```python
from build123d import *

# Parameters (mm, degrees)
BOSS_EXTRUDE1_DEPTH   = 1.5875
SKETCH3_R             = 4.445
SKETCH3_W             = 12.065
SKETCH3_H             = 12.065
CUT_EXTRUDE1_DEPTH    = 2.5875
SKETCH4_R             = 3.96875
CUT_EXTRUDE2_DEPTH    = 2.5875
SKETCH5_W             = 11.94
SKETCH5_H             = 20.64
SKETCH5_W_2           = 45.462
SKETCH5_H_2           = 102.32
SKETCH5_W_3           = 57
SKETCH5_H_3           = 15.1
CUT_EXTRUDE3_DEPTH    = 2.5875
F_6_CLEARANCE_HOLE2_D = 4.3053
CUT_EXTRUDE4_START    = -1.5875
SKETCH11_W            = 13.529020254
SKETCH11_H            = 14.424558238
SKETCH11_W_2          = 13.332833864
SKETCH11_H_2          = 14.312726797
CUT_EXTRUDE4_DEPTH    = 1.5875


with BuildPart() as part:
    # Sketch1 → Boss-Extrude1 (new body)
    with BuildSketch(Plane.XY):
        with BuildLine():
            Line((74.93, -171.1167297), (86.51875, -171.1167297))
            Line((86.51875, -171.1167297), (86.51875, -67.9292297))
            Line((86.51875, -67.9292297), (-86.51875, -67.9292297))
            Line((-86.51875, -67.9292297), (-86.51875, -171.1167297))
            Line((-86.51875, -171.1167297), (-74.93, -171.1167297))
            ThreePointArc((-74.93, -171.1167297), (-71.337897552, -172.604627251), (-69.85, -176.1967297))
            Line((-69.85, -176.1967297), (-69.85, -182.2292297))
            Line((-69.85, -182.2292297), (69.85, -182.2292297))
            Line((69.85, -182.2292297), (69.85, -176.1967297))
            ThreePointArc((69.85, -176.1967297), (71.337897552, -172.604627251), (74.93, -171.1167297))
        make_face()
    extrude(amount=-BOSS_EXTRUDE1_DEPTH)

    # Sketch3 → Cut-Extrude1 (cut, through all)
    with BuildSketch(Plane.XY):
        with Locations((74.93, -159.3692297)):
            Circle(SKETCH3_R)
        with Locations((-6.731, -165.7192297)):
            Circle(SKETCH3_R)
        with Locations((-6.731, -145.3992297)):
            Circle(SKETCH3_R)
        with Locations((-6.731, -125.0792297)):
            Circle(SKETCH3_R)
        with Locations((-6.731, -104.7592297)):
            Circle(SKETCH3_R)
        with Locations((-6.731, -84.4392297)):
            Circle(SKETCH3_R)
        with Locations((-73.66, -139.0492297)):
            Rectangle(SKETCH3_W, SKETCH3_H)
        with Locations((13.843, -143.3672297)):
            Rectangle(SKETCH3_W, SKETCH3_H)
        with Locations((32.639, -143.3672297)):
            Rectangle(SKETCH3_W, SKETCH3_H)
        with Locations((51.435, -143.3672297)):
            Rectangle(SKETCH3_W, SKETCH3_H)
        with Locations((51.435, -124.5712297)):
            Rectangle(SKETCH3_W, SKETCH3_H)
        with Locations((32.639, -124.5712297)):
            Rectangle(SKETCH3_W, SKETCH3_H)
        with Locations((13.843, -124.5712297)):
            Rectangle(SKETCH3_W, SKETCH3_H)
        with Locations((13.843, -105.7752297)):
            Rectangle(SKETCH3_W, SKETCH3_H)
        with Locations((13.843, -86.9792297)):
            Rectangle(SKETCH3_W, SKETCH3_H)
        with Locations((32.639, -86.9792297)):
            Rectangle(SKETCH3_W, SKETCH3_H)
        with Locations((32.639, -105.7752297)):
            Rectangle(SKETCH3_W, SKETCH3_H)
        with Locations((51.435, -105.7752297)):
            Rectangle(SKETCH3_W, SKETCH3_H)
        with Locations((51.435, -86.9792297)):
            Rectangle(SKETCH3_W, SKETCH3_H)
    extrude(amount=-CUT_EXTRUDE1_DEPTH, mode=Mode.SUBTRACT)

    # Sketch4 → Cut-Extrude2 (cut, through all)
    with BuildSketch(Plane.XY):
        with Locations((-73.025, -113.9667297)):
            Circle(SKETCH4_R)
        with Locations((-73.025, -159.0517297)):
            Circle(SKETCH4_R)
        with Locations((74.295, -113.9667297)):
            Circle(SKETCH4_R)
        with Locations((75.184, -139.0492297)):
            Circle(SKETCH4_R)
    extrude(amount=-CUT_EXTRUDE2_DEPTH, mode=Mode.SUBTRACT)

    # Sketch5 → Cut-Extrude3 (cut, through all)
    with BuildSketch(Plane.XY):
        with Locations((-73.66, -84.3122297)):
            Rectangle(SKETCH5_W, SKETCH5_H)
        with Locations((73.66, -84.3122297)):
            Rectangle(SKETCH5_W, SKETCH5_H)
        with Locations((-39.799, -124.9522297)):
            Rectangle(SKETCH5_W_2, SKETCH5_H_2)
        with Locations((33.02, -165.4922297)):
            Rectangle(SKETCH5_W_3, SKETCH5_H_3)
    extrude(amount=-CUT_EXTRUDE3_DEPTH, mode=Mode.SUBTRACT)

    # #6 Clearance Hole2 (through all)
    with Locations(Plane(origin=(0, 0, 0), x_dir=(-1, 0, 0), z_dir=(0, 0, 1))):
        with Locations((-81.28, 124.6982297), (6.731, 175.8792297), (81.28, 124.6982297), (6.731, 74.2792297)):
            Hole(F_6_CLEARANCE_HOLE2_D / 2)

    # Sketch11 → Cut-Extrude4 (cut)
    with BuildSketch(Plane(origin=(0, 0, -1.5875), x_dir=(-1, 0, 0), z_dir=(0, 0, -1)).offset(CUT_EXTRUDE4_START)):
        with Locations((73.612537257, -84.279184845)):
            Rectangle(SKETCH11_W, SKETCH11_H)
        with Locations((-73.648214967, -84.336507402)):
            Rectangle(SKETCH11_W_2, SKETCH11_H_2)
    extrude(amount=CUT_EXTRUDE4_DEPTH, mode=Mode.SUBTRACT)


solid = part.part
```
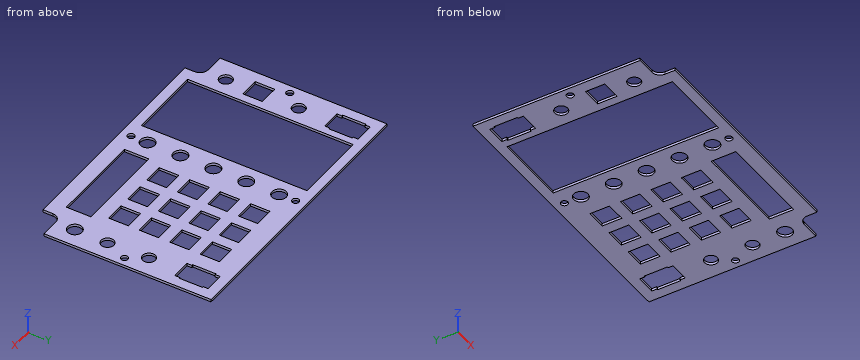
Geometry: final body of the model. Coordinates: model frame, mm. Round coordinates to 2 decimals unless told otherwise and drop trailing zeros. Order: outer loops, then holes, each group sorted by start corner. A loop starts at its lowest first (then second) coordinate and runs counter-clockwise, first axis right, second up. Notation, with made-up numbers: (-20, 4.5) -> (13, 4.5) arc R24 ccw to (13, 40.5) -> close; hole circle Ø1 at (43, -9). An arc over 180 degrees is marked (long way). Use CSV: the item, a comma, the result in double quotes. Start each with the question number.
1) Section D-D (z = -0.9). State how many separate pieces and enclosed holes the cut face has, and give its area (3 significant figures).
2) Section C-C (y = -168). Return the cut outline in (x, z), and give its area (3 significant figures).
3) Section A-A (x = -60.5). Return the cut outline in (y, z), and give its area (3 significant figures).
4) First-contact query: pin 1 Ø8 at (x, y) = (-6.73, -165.72) entering from -Z; pin 2 Ø0.8 at (y, z) = (-178, -0.5) entering from +X; pin 3 Ø0.5 at (x, z) = (-73, -1) entering from -Y. Flat tips, straight axial feed; report the tip coordinate or a pass-through.
5) Material intervals for line 1 along X through (y, z) = (-171, -0.25); line 2 along X through (y, z) = (-109.5, -0.1); line 3 along Y through (x, z) = (53.5, -1.05), sorted ascending. Write a range as from..to.
6) Section B-B (x = 36). Return the cut outline in (y, z), and give its area (3 significant figures).
Returned:
1,separate pieces,"1"
1,enclosed holes,"31"
1,area,"10,800 mm²"
2,outline,"(-86.52, -1.59) -> (-62.53, -1.59) -> (-62.53, 0) -> (-86.52, 0) -> close; (-17.07, -1.59) -> (-10.55, -1.59) -> (-10.55, 0) -> (-17.07, 0) -> close; (-2.92, -1.59) -> (4.52, -1.59) -> (4.52, 0) -> (-2.92, 0) -> close; (61.52, -1.59) -> (86.52, -1.59) -> (86.52, 0) -> (61.52, 0) -> close"
2,area,"99.9 mm²"
3,outline,"(-182.23, -1.59) -> (-176.11, -1.59) -> (-176.11, 0) -> (-182.23, 0) -> close; (-73.79, -1.59) -> (-67.93, -1.59) -> (-67.93, 0) -> (-73.79, 0) -> close"
3,area,"19.0 mm²"
4,pin 1,"passes through"
4,pin 2,"stops at x = 69.85"
4,pin 3,"stops at y = -171.61"
5,line 1,"x = -86.52..-62.53, -17.07..4.52, 61.52..86.52"
5,line 2,"x = -86.52..-62.53, -17.07..7.81, 19.88..26.61, 38.67..45.4, 57.47..86.52"
5,line 3,"y = -182.23..-173.04, -157.94..-149.4, -137.33..-130.6, -118.54..-111.81, -99.74..-93.01, -80.95..-67.93"
6,outline,"(-182.23, -1.59) -> (-173.04, -1.59) -> (-173.04, 0) -> (-182.23, 0) -> close; (-157.94, -1.59) -> (-149.4, -1.59) -> (-149.4, 0) -> (-157.94, 0) -> close; (-137.33, -1.59) -> (-130.6, -1.59) -> (-130.6, 0) -> (-137.33, 0) -> close; (-118.54, -1.59) -> (-111.81, -1.59) -> (-111.81, 0) -> (-118.54, 0) -> close; (-99.74, -1.59) -> (-93.01, -1.59) -> (-93.01, 0) -> (-99.74, 0) -> close; (-80.95, -1.59) -> (-67.93, -1.59) -> (-67.93, 0) -> (-80.95, 0) -> close"
6,area,"80.9 mm²"
